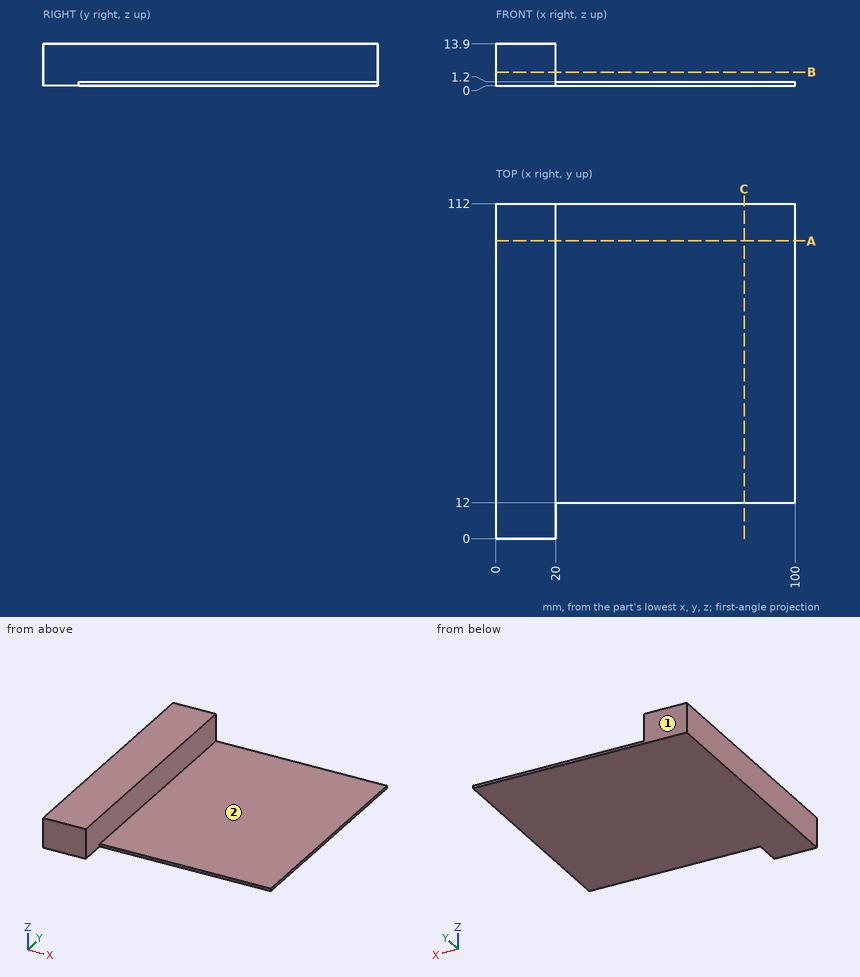
Could you check a few things on this drawing? It's one solid part, dimensions in mm from its lowest x, y, z. A direction names the side the tool comes from. Give positions to 0.01 mm unless a question says otherwise; leave off trailing zeros. Order: outer loops, then holes, each group sorted by start corner. A loop starts at its lowest first (then second) coordinate and runs counter-clockwise, first axis right, second up. Notation, with made-up numbers: (41.5, 35.5) -> (90.5, 35.5) arc R5 cw to (90.5, 40.5) -> close; hole circle Ø9 at (78, 30.25). An arc over 180 degrees is marked (long way). Use CSV: the item, a comma, the result in double quotes. Start each with the question number.
Item 1: Suppose I cut it at B-B (z = 4.5). List the corners of the cut face in (x, y) for me.
Item 2: Suppose I cut it at C-C (x = 83). List the corners of the cut face in (y, z) for me.
Item 3: If I drill on probe 1 along Z at (x, y) = (26, 104); probe 2 along X at (y, z) = (16, 5.5); probe 3 along Y at (x, z) = (67.5, 0.5), over which ranges is the centre line in solid material (lowest first)? Write a range as [from, to].
Item 4: On a 3-axis mill with a long thin cutter (end or side, diameter ignored), from which of +Z, -Z, +X, -X, +Y, -Y can I reach the whole of each face in a straight line? I mean the marked faces 1 and 2. Say none if no direction works.
Item 5: Suppose I cut it at A-A (y = 99.5). List the corners of the cut face in (x, z) for me, and give its area (3 significant figures).
Item 6: I'm going to push flat-ended pins straight in: P1, Ø1, axis at x = 68, z = 0.5, coming from the -Y side; P2, Ø4, axis at y = 64, z = 10, coming from the +X side. Where does each tip first touch, or does it pass through?
Answer block:
1,outline,"(0, 0) -> (20, 0) -> (20, 112) -> (0, 112) -> close"
2,outline,"(12, 0) -> (112, 0) -> (112, 1.2) -> (12, 1.2) -> close"
3,probe 1,"z = [0, 1.2]"
3,probe 2,"x = [0, 20]"
3,probe 3,"y = [12, 112]"
4,face 1,"+Z, -Z, +X, -X, +Y"
4,face 2,"+Z, +X, +Y, -Y"
5,outline,"(0, 0) -> (100, 0) -> (100, 1.2) -> (20, 1.2) -> (20, 13.9) -> (0, 13.9) -> close"
5,area,"374 mm^2"
6,P1,"stops at y = 12"
6,P2,"stops at x = 20"
